```python
from build123d import *

# Parameters (mm, degrees)
BOSS_EXTRUDE1_DEPTH      = 60
BOSS_EXTRUDE1_DEPTH_BACK = 60
SKETCH1_W                = 114
SKETCH1_H                = 16
SKETCH2_W                = 108
SKETCH2_H                = 26
CUT_EXTRUDE1_DEPTH       = 134.090194981


with BuildPart() as part:
    # Sketch1 → Boss-Extrude1 (new, two sides: drawn at the far end of the back side and taken through both)
    with BuildSketch(Plane.XY.offset(-BOSS_EXTRUDE1_DEPTH_BACK)):
        Rectangle(SKETCH1_W, SKETCH1_H)
    extrude(amount=BOSS_EXTRUDE1_DEPTH + BOSS_EXTRUDE1_DEPTH_BACK)

    # Sketch2 → Cut-Extrude1 (cut, through all)
    with BuildSketch(Plane.XY.offset(60)):
        with Locations((0, 8)):
            Rectangle(SKETCH2_W, SKETCH2_H)
    extrude(amount=-CUT_EXTRUDE1_DEPTH, mode=Mode.SUBTRACT)


solid = part.part
```
Verification items for the finished model (mm, model axes). A direction names the side the tool comes from. Round coordinates to 2 decimals unless told otherwise and drop trailing zeros. Write each loop counter-clockwise with the first axis right and the second up, starting at its lowest first coordinate (ties: lowest second). Pieces come first, ordered by that corner, then holes.
1. Gauge pin test, flat end, axial feed: P1, Ø10, axis at x = -44, z = 31.5, coming from the +Y side. Record the tip position at first contact, or that the pin passes through.
2. Access from +Z, -Z, +X, -X, +Y, -Y to the whole of each face (thin tool, end or side, straight path). Record for faces 5 (the flat face through (-56, 8, -1)), 6 (the flat face through (-1, -5, 1)).
3. Section check C-C on x = -46. Enter the section's corners in (y, z).
4. Scan lines: L1, parallel to X at y = 1, z = 14.5; L2, parallel to Y at x = -16.5, z = 40. Record each from-to range of solid material in increasing order.
5. Section check B-B on z = 44. Enter the section's corners in (x, y), plus the area to 3 significant figures.
6. Draft check along X on faces 1 (the flat face through (-54, 1, 1)), 2 (the flat face through (55, 8, -1)), 3 (the flat face through (57, 0, -1)), 4 (the flat face through (54, 1, 1)). Enter one of: +X half, -X half, draft (parallel to the pull), parting line (faces both ways), or undercut.
7. Section check A-A on y = 1.5. Enter the section's corners in (x, z).
Answer:
1. P1: stops at y = -5
2. face 5: +Z, -Z, +X, -X, +Y
2. face 6: +Z, -Z, +Y
3. outline: (-8, -60) - (-5, -60) - (-5, 60) - (-8, 60) - close
4. L1: x = -57 to -54, 54 to 57
4. L2: y = -8 to -5
5. outline: (-57, -8) - (57, -8) - (57, 8) - (54, 8) - (54, -5) - (-54, -5) - (-54, 8) - (-57, 8) - close
5. area: 420 mm2
6. face 1: undercut
6. face 2: draft
6. face 3: +X half
6. face 4: undercut
7. outline: (-57, -60) - (-54, -60) - (-54, 60) - (-57, 60) - close; (54, -60) - (57, -60) - (57, 60) - (54, 60) - close
